from build123d import *

# Parameters (mm, degrees)
BOSS_EXTRUDE1_DEPTH = 2
CUT_EXTRUDE1_DEPTH  = 104.743351649
SKETCH4_W           = 67.1
SKETCH4_H           = 9
BOSS_EXTRUDE2_DEPTH = 2


with BuildPart() as part:
    # Sketch2 → Boss-Extrude1 (new body)
    with BuildSketch(Plane.XY):
        Polygon((-88.945731411, -6.4), (-88.945731411, -1.9), (-93.645731411, -1.9), (-93.645731411, -44.6), (-26.145731411, -44.6), (-26.145731411, -1.9), (-70.145731411, -1.9), (-70.145731411, -6.4), align=None)
    extrude(amount=BOSS_EXTRUDE1_DEPTH)

    # Sketch3 → Cut-Extrude1 (cut, through all)
    with BuildSketch(Plane.XY.offset(2)):
        Polygon((-88.945731411, -1.9), (-93.645731411, -1.9), (-93.645731411, -44.6), (-26.145731411, -44.6), (-26.145731411, -1.9), (-70.145731411, -1.9), (-70.145731411, -6.4), (-88.945731411, -6.4), align=None)
        Polygon((-89.145731411, -2.1), (-93.445731411, -2.1), (-93.445731411, -44.4), (-26.345731411, -44.4), (-26.345731411, -2.1), (-69.945731411, -2.1), (-69.945731411, -6.6), (-89.145731411, -6.6), align=None, mode=Mode.SUBTRACT)
    extrude(amount=-CUT_EXTRUDE1_DEPTH, mode=Mode.SUBTRACT)

    # Sketch4 → Boss-Extrude2 (add)
    with BuildSketch(Plane.XY.offset(2)):
        with Locations((-59.895731411, -48.9)):
            Rectangle(SKETCH4_W, SKETCH4_H)
    extrude(amount=-BOSS_EXTRUDE2_DEPTH)


solid = part.part
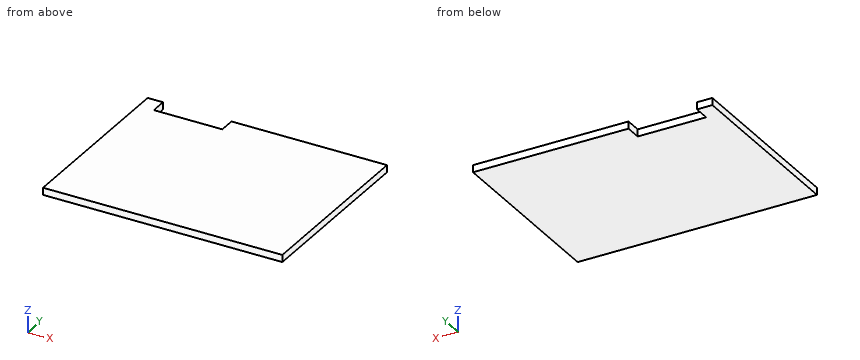
CAD build for the part. Positions are in the model's coordinates, mm. Round coordinates to 2 decimals unless told otherwise and drop trailing zeros. Loops run counter-clockwise (first coordinate to the right, second up) from the corner with the lowest first, then second, coordinate; pieces in that order, holes last.
(1) Cut at B-B (x = -87). Give the cut face in (y, z).
(2) Wall check: line 1 along X through (y, z) = (-6, 0.45); line 2 along Y through (x, z) = (-78, 1). Give the ranges that are in metal, low to high.
(3) Cut at A-A (z = 1.7). Give the cut face in (x, y).
(4) Drop a flat-ended pin along its axis: pin 1 (1 mm diameter, centred on x = -80, z = 1, fed in from +Y). Give the stop position or say it passes through.
Findings below:
1. outline: (-53.4, 0) - (-6.6, 0) - (-6.6, 2) - (-53.4, 2) - close
2. line 1: x = -93.45 to -89.15, -69.95 to -26.35
2. line 2: y = -53.4 to -6.6
3. outline: (-93.45, -53.4) - (-26.35, -53.4) - (-26.35, -2.1) - (-69.95, -2.1) - (-69.95, -6.6) - (-89.15, -6.6) - (-89.15, -2.1) - (-93.45, -2.1) - close
4. pin 1: stops at y = -6.6
